Geometry check sheet. Reference: drawing and pictorial views, mm from the part's lowest x, y, z. A direction names the side the tool comes from. Round coordinates to 2 decimals unless told otherwise and drop trailing zeros. Write each loop counter-clockwise with the first axis right and the second up, starting at its lowest first coordinate (ties: lowest second). Pieces come first, ordered by that corner, then holes.
Item 1: Section check B-B, the plane x = 12. Record the cut outline in (y, z) (1 decimal).
Item 2: Release check for a two-part mould opening along Y. For the marked faces 3, 4 and 5 record: pulls with the +Y half, pulls with the -Y half, needs draft (parallel to the pull), parting line crosses it, or undercut.
Item 3: Material ranges on line 1 along Y through (x, z) = (20, 8); line 2 along X through (y, z) = (2, 7.75); line 3 along Z through (x, y) = (1.75, 8), recorded low to high.
Item 4: Section check C-C, the plane y = 6.25. Record the cut outline in (x, z).
Item 5: Section check D-D, the plane y = 4. Record the cut outline in (x, z) (1 decimal).
Item 6: Set-up check for the marked faces 1 and 2: record each of +Z, -Z, +X, -X, +Y, -Y from which the full face is reachable in a straight line by a thin tool's end or side.
Item 7: Depth check by flat-ended pin: pin 1 (5 mm diameter, centred on x = 14, y = 1, fed in from -Z); pin 2 (2 mm diameter, centred on x = 7.5, y = 4, fed in from +Z). Enter the tip coordinate at first touch or a pass-through.
Item 8: Section check A-A, the plane z = 6.25. Record the cut outline in (x, y).
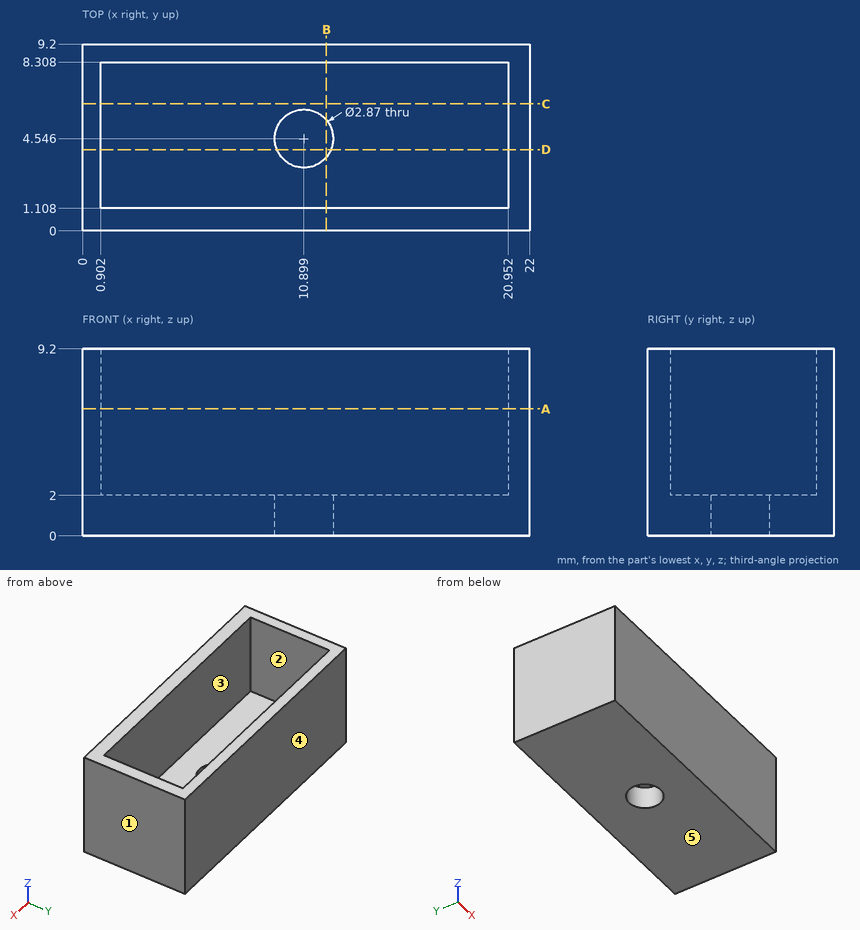
Values found:
1. outline: (0, 0) - (3.6, 0) - (3.6, 2) - (1.1, 2) - (1.1, 9.2) - (0, 9.2) - close; (5.5, 0) - (9.2, 0) - (9.2, 9.2) - (8.3, 9.2) - (8.3, 2) - (5.5, 2) - close
2. face 3: undercut
2. face 4: pulls with the +Y half
2. face 5: needs draft
3. line 1: y = 0 to 1.11, 8.31 to 9.2
3. line 2: x = 0 to 0.9, 20.95 to 22
3. line 3: z = 0 to 2
4. outline: (0, 0) - (22, 0) - (22, 9.2) - (20.95, 9.2) - (20.95, 2) - (0.9, 2) - (0.9, 9.2) - (0, 9.2) - close
5. outline: (0, 0) - (9.6, 0) - (9.6, 2) - (0.9, 2) - (0.9, 9.2) - (0, 9.2) - close; (12.2, 0) - (22, 0) - (22, 9.2) - (21, 9.2) - (21, 2) - (12.2, 2) - close
6. face 1: +Z, -Z, +X, +Y, -Y
6. face 2: +Z
7. pin 1: stops at z = 0
7. pin 2: stops at z = 2
8. outline: (0, 0) - (22, 0) - (22, 9.2) - (0, 9.2) - close; hole (0.9, 1.11) - (20.95, 1.11) - (20.95, 8.31) - (0.9, 8.31) - close
